Drawing for the job (mm, zero at the part's lowest x, y, z). Coordinates: 2 decimals unless noted, no trailing zeros. Order: outer loops, then holes, each group sorted by start corner. A loop starts at its lowest first (then second) coordinate and runs counter-clockwise, first axis right, second up.
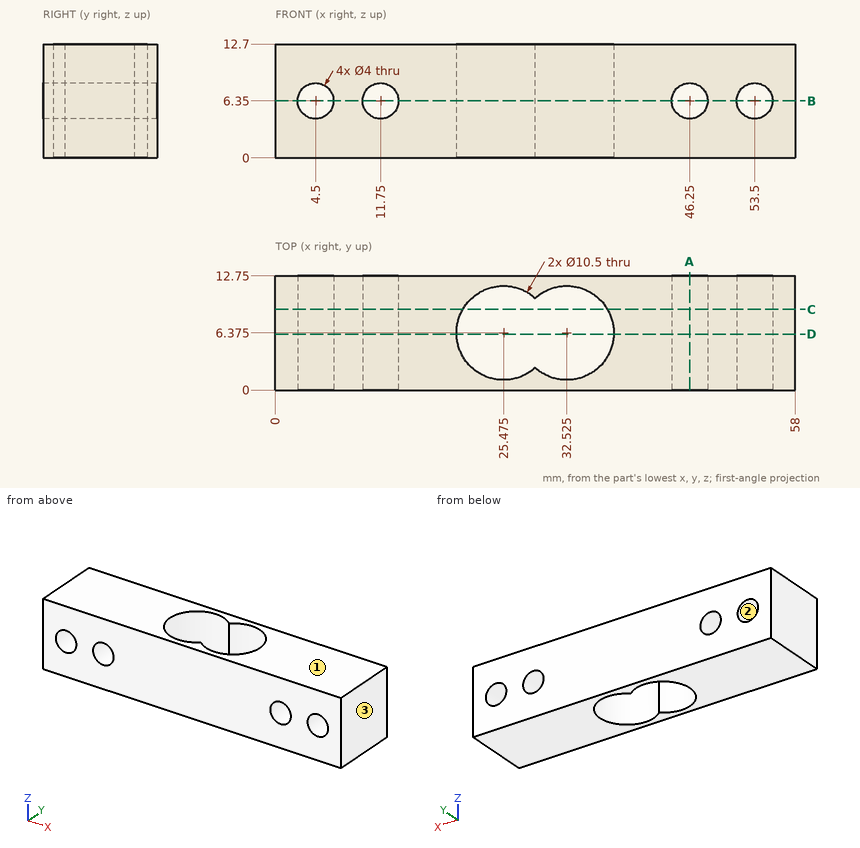
(1) Pull direction Z, two halves, no side cores. Call the marked faces 1, 2 and 3: +Z half, -Z half, draft (parallel to the pull), parting line (faces both ways), or undercut.
(2) Slice it at B-B, the plane z = 6.35. Give the cut face in (x, y) (3 decimals), then the cut area to 3 significant figures.
(3) Slice it at C-C, the plane y = 9. Give the cut face in (x, z), then the cut area to 3 significant figures.
(4) Slice it at A-A, the plane x = 46.25. Give the cut face in (y, z).
(5) Slice it at D-D, the plane y = 6.25. Give the cut face in (x, z).
(6) Probe line 1 (X direction, y = 6.75, z = 5.75); line 2 (X direction, y = 3, z = 6.35); line 3 (X direction, y = 6.5, z = 9). List the from-to ranges inside material, lowest first.
Here are the results:
1. face 1: +Z half
1. face 2: undercut
1. face 3: draft
2. outline: (0, 0) - (2.5, 0) - (2.5, 12.75) - (0, 12.75) - close; (6.5, 0) - (9.75, 0) - (9.75, 12.75) - (6.5, 12.75) - close; (13.75, 0) - (44.25, 0) - (44.25, 12.75) - (13.75, 12.75) - close; (48.25, 0) - (51.5, 0) - (51.5, 12.75) - (48.25, 12.75) - close; (55.5, 0) - (58, 0) - (58, 12.75) - (55.5, 12.75) - close; hole (29, 2.484) arc R5.25 ccw (long way) to (29, 10.266) arc R5.25 ccw (long way) to start
2. area: 381 mm2
3. outline: (0, 0) - (20.93, 0) - (20.93, 12.7) - (0, 12.7) - close; (37.07, 0) - (58, 0) - (58, 12.7) - (37.07, 12.7) - close; hole circle Ø4 at (4.5, 6.35); hole circle Ø4 at (11.75, 6.35); hole circle Ø4 at (46.25, 6.35); hole circle Ø4 at (53.5, 6.35)
3. area: 481 mm2
4. outline: (0, 0) - (12.75, 0) - (12.75, 4.35) - (0, 4.35) - close; (0, 8.35) - (12.75, 8.35) - (12.75, 12.7) - (0, 12.7) - close
5. outline: (0, 0) - (20.23, 0) - (20.23, 12.7) - (0, 12.7) - close; (37.77, 0) - (58, 0) - (58, 12.7) - (37.77, 12.7) - close; hole circle Ø4 at (4.5, 6.35); hole circle Ø4 at (11.75, 6.35); hole circle Ø4 at (46.25, 6.35); hole circle Ø4 at (53.5, 6.35)
6. line 1: x = 0 to 2.59, 6.41 to 9.84, 13.66 to 20.24, 37.76 to 44.34, 48.16 to 51.59, 55.41 to 58
6. line 2: x = 0 to 2.5, 6.5 to 9.75, 13.75 to 21.45, 36.55 to 44.25, 48.25 to 51.5, 55.5 to 58
6. line 3: x = 0 to 20.23, 37.77 to 58
